Geometry: final body of the model. Coordinates: model frame, mm. A direction names the side the tool comes from. Round coordinates to 2 decimals unless told otherwise and drop trailing zeros. Loops run counter-clockwise (first coordinate to the right, second up) from the corner with the lowest first, then second, coordinate; pieces in that order, holes last. Notation, with made-up numbers: M 89.5,19 L 134.5,19 A22 ccw 134.5,51 Z; hole C -9,54 d8. An arc over 180 degrees is marked long. Write each question's results on one line, items separated by ' | '.
```python
from build123d import *

# Parameters (mm, degrees)
F1_DEPTH = 110
F3_DEPTH = 6.35
F4_R     = 3.175
F5_DEPTH = 25.4


with BuildPart() as f1:
    # F0 (on Top) → F1 (new body)
    with BuildSketch(Plane.XY):
        with BuildLine():
            ThreePointArc((14, 72.46), (13.256051, 74.256051), (11.46, 75))
            Line((11.46, 75), (-11.46, 75))
            ThreePointArc((-11.46, 75), (-13.256051, 74.256051), (-14, 72.46))
            Line((-14, 72.46), (-14, -72.46))
            ThreePointArc((-14, -72.46), (-13.256051, -74.256051), (-11.46, -75))
            Line((-11.46, -75), (11.46, -75))
            ThreePointArc((11.46, -75), (13.256051, -74.256051), (14, -72.46))
            Line((14, -72.46), (14, 72.46))
        make_face()
    extrude(amount=F1_DEPTH)

    # F2 (on face) → F3 (join)
    with BuildSketch(Plane.XY.offset(110)):
        with BuildLine():
            ThreePointArc((-11.46, -66.11), (-10.716051, -67.906051), (-8.92, -68.65))
            Line((-8.92, -68.65), (8.92, -68.65))
            ThreePointArc((8.92, -68.65), (10.716051, -67.906051), (11.46, -66.11))
            Line((11.46, -66.11), (11.46, -30.48))
            ThreePointArc((11.46, -30.48), (10.716051, -28.683949), (8.92, -27.94))
            Line((8.92, -27.94), (-8.92, -27.94))
            ThreePointArc((-8.92, -27.94), (-10.716051, -28.683949), (-11.46, -30.48))
            Line((-11.46, -30.48), (-11.46, -66.11))
        make_face()
        with BuildLine():
            Line((8.92, 68.65), (-8.92, 68.65))
            ThreePointArc((-8.92, 68.65), (-10.716051, 67.906051), (-11.46, 66.11))
            Line((-11.46, 66.11), (-11.46, 30.48))
            ThreePointArc((-11.46, 30.48), (-10.716051, 28.683949), (-8.92, 27.94))
            Line((-8.92, 27.94), (8.92, 27.94))
            ThreePointArc((8.92, 27.94), (10.716051, 28.683949), (11.46, 30.48))
            Line((11.46, 30.48), (11.46, 66.11))
            ThreePointArc((11.46, 66.11), (10.716051, 67.906051), (8.92, 68.65))
        make_face()
    extrude(amount=F3_DEPTH)

    # F4 (on face) → F5 (join)
    with BuildSketch(Plane.XY.offset(116.35)):
        with Locations((0, -37.465)):
            Circle(F4_R)
        with Locations((0, 37.465)):
            Circle(F4_R)
    extrude(amount=F5_DEPTH)


solid = f1.part
```
1. Section C-C (x = -5.5). Output: boundary loops of the cut face in (y, z).
Answer key:
outline: M -75,0 L 75,0 L 75,110 L 68.65,110 L 68.65,116.35 L 27.94,116.35 L 27.94,110 L -27.94,110 L -27.94,116.35 L -68.65,116.35 L -68.65,110 L -75,110 Z
2. Section B-B (z = 114). Output: boundary loops of the cut face in (x, y), then the cut area to 3 significant figures.
Answer key:
outline: M -11.46,-66.11 A2.54 ccw -8.92,-68.65 L 8.92,-68.65 A2.54 ccw 11.46,-66.11 L 11.46,-30.48 A2.54 ccw 8.92,-27.94 L -8.92,-27.94 A2.54 ccw -11.46,-30.48 Z; M -11.46,30.48 A2.54 ccw -8.92,27.94 L 8.92,27.94 A2.54 ccw 11.46,30.48 L 11.46,66.11 A2.54 ccw 8.92,68.65 L -8.92,68.65 A2.54 ccw -11.46,66.11 Z | area: 1,860 mm²
3. Access query for faces 4 (the face through (0, 1, 110)), 5 (the face through (0, -68.65, 113)), 6 (the face through (-11.46, -48, 113)). Directions: +Z, -Z, +X, -X, +Y, -Y. A direction counts if a zero-diameter tool reaches every point of the face in a straight line with its end or side. Return the directions, or none.
Answer key:
face 4: +Z | face 5: +Z, +X, -X, -Y | face 6: +Z, -X, +Y, -Y
4. Pin query (flat end, axial travel): P1, Ø7, axis at x = -5, y = -54.5, coming from the +Z side; P2, Ø3, axis at y = 53, z = 112, coming from the +X side; P3, Ø1.5, axis at x = 8.5, z = 117, coming from the +Y side. Return the tip coordinate at first contact, or that it passes through.
Answer key:
P1: stops at z = 116.35 | P2: stops at x = 11.46 | P3: stops at y = 68.65
5. Section A-A (y = 49.5). Output: boundary loops of the cut face in (x, z), then the cut area to 3 significant figures.
Answer key:
outline: M -14,0 L 14,0 L 14,110 L 11.46,110 L 11.46,116.35 L -11.46,116.35 L -11.46,110 L -14,110 Z | area: 3,230 mm²
6. Draft query along Y for faces 1 (the face through (0, 68.65, 113)), 2 (the face through (0, 27.94, 113)), 3 (the face through (-11.46, 49, 113)). Return one class per face: pulls with the +Y half, pulls with the -Y half, needs draft (parallel to the pull), parting line crosses it, or undercut.
Answer key:
face 1: pulls with the +Y half | face 2: undercut | face 3: needs draft
7. Section D-D (y = -9). Output: boundary loops of the cut face in (x, z).
Answer key:
outline: M -14,0 L 14,0 L 14,110 L -14,110 Z
8. Ray query, probe 1 along Z at (x, y) = (-1.75, -26); probe 2 along X at (y, z) = (66, 114.5); probe 3 along Z at (x, y) = (-8, 59). Return the intervals inside material, ascending.
Answer key:
probe 1: z = 0 to 110 | probe 2: x = -11.46 to 11.46 | probe 3: z = 0 to 116.35
